from build123d import *

# Parameters (mm, degrees)
CROQUIS1_W              = 3
CROQUIS1_H              = 3
SALIENTE_EXTRUIR1_DEPTH = 6
CROQUIS2_R              = 0.65
SALIENTE_EXTRUIR2_DEPTH = 3.5
SALIENTE_EXTRUIR3_START = 2
CROQUIS6_R              = 0.65
SALIENTE_EXTRUIR3_DEPTH = 2


with BuildPart() as part:
    # Croquis1 → Saliente-Extruir1 (new body)
    with BuildSketch(Plane(origin=(0, 0, 0), x_dir=(0, 0, -1), z_dir=(1, 0, 0))):
        with Locations((0, 0.5)):
            Rectangle(CROQUIS1_W, CROQUIS1_H)
    extrude(amount=SALIENTE_EXTRUIR1_DEPTH)

    # Croquis2 → Saliente-Extruir2 (add)
    with BuildSketch(Plane.ZY):
        with Locations(Location((0, 0.5, 0), (0, 0, 180))):
            Circle(CROQUIS2_R)
    extrude(amount=SALIENTE_EXTRUIR2_DEPTH)

    # Croquis6 → Saliente-Extruir3 (add)
    with BuildSketch(Plane(origin=(6, 0, 0), x_dir=(0, 0, -1), z_dir=(1, 0, 0)).offset(SALIENTE_EXTRUIR3_START)):
        with Locations((0, 0.5)):
            Circle(CROQUIS6_R)
    extrude(amount=-SALIENTE_EXTRUIR3_DEPTH)


solid = part.part
Geometry: final body of the model. Coordinates: model frame, mm. A direction names the side the tool comes from. Coordinates: 2 decimals unless noted, no trailing zeros. Order: outer loops, then holes, each group sorted by start corner. A loop starts at its lowest first (then second) coordinate and runs counter-clockwise, first axis right, second up.
(1) Section query D-D (y = -0.4). Return the cut outline in (x, z), plus the area to 3 significant figures.
(2) Material intervals for probe 1 along X at (y, z) = (0.1, -1.15); probe 2 along Z at (x, y) = (-1.25, 1.05); probe 3 along Y at (x, z) = (-2.5, 0.5), sorted ascending.
(3) Section query C-C (x = -0.25). Return the cut outline in (y, z), plus the area to 3 significant figures.
(4) Section query A-A (y = 0.5). Return the cut outline in (x, z), plus the area to 4 significant figures.
(5) Access query for faces 1 (the face through (6, 1, 1)), 2 (the face through (0, 1, 1)), 3 (the face through (8, 0.5, 0)). Directions: +Z, -Z, +X, -X, +Y, -Y. A direction counts if a zero-diameter tool reaches every point of the face in a straight line with its end or side. Return the directions, or none.
(6) Section query B-B (z = 0). Return the cut outline in (x, y).
(7) Draft query along Y for faces 4 (the face through (3, -1, 0)), 5 (the face through (-1.726, 0.896, 0.516)), 6 (the face through (3, 2, 0)), 7 (the face through (3, 0, -1.5)). Return one class per face: pulls with the +Y half, pulls with the -Y half, needs draft (parallel to the pull), parting line crosses it, or undercut.
Solution:
1. outline: (0, -1.5) - (6, -1.5) - (6, 1.5) - (0, 1.5) - close
1. area: 18.0 mm2
2. probe 1: x = 0 to 6
2. probe 2: z = -0.35 to 0.35
2. probe 3: y = 0.08 to 0.92
3. outline: circle Ø1.3 at (0.5, 0)
3. area: 1.33 mm2
4. outline: (-3.5, -0.65) - (0, -0.65) - (0, -1.5) - (6, -1.5) - (6, -0.65) - (8, -0.65) - (8, 0.65) - (6, 0.65) - (6, 1.5) - (0, 1.5) - (0, 0.65) - (-3.5, 0.65) - close
4. area: 25.15 mm2
5. face 1: +X
5. face 2: -X
5. face 3: +Z, -Z, +X, +Y, -Y
6. outline: (-3.5, -0.15) - (0, -0.15) - (0, -1) - (6, -1) - (6, -0.15) - (8, -0.15) - (8, 1.15) - (6, 1.15) - (6, 2) - (0, 2) - (0, 1.15) - (-3.5, 1.15) - close
7. face 4: pulls with the -Y half
7. face 5: parting line crosses it
7. face 6: pulls with the +Y half
7. face 7: needs draft
